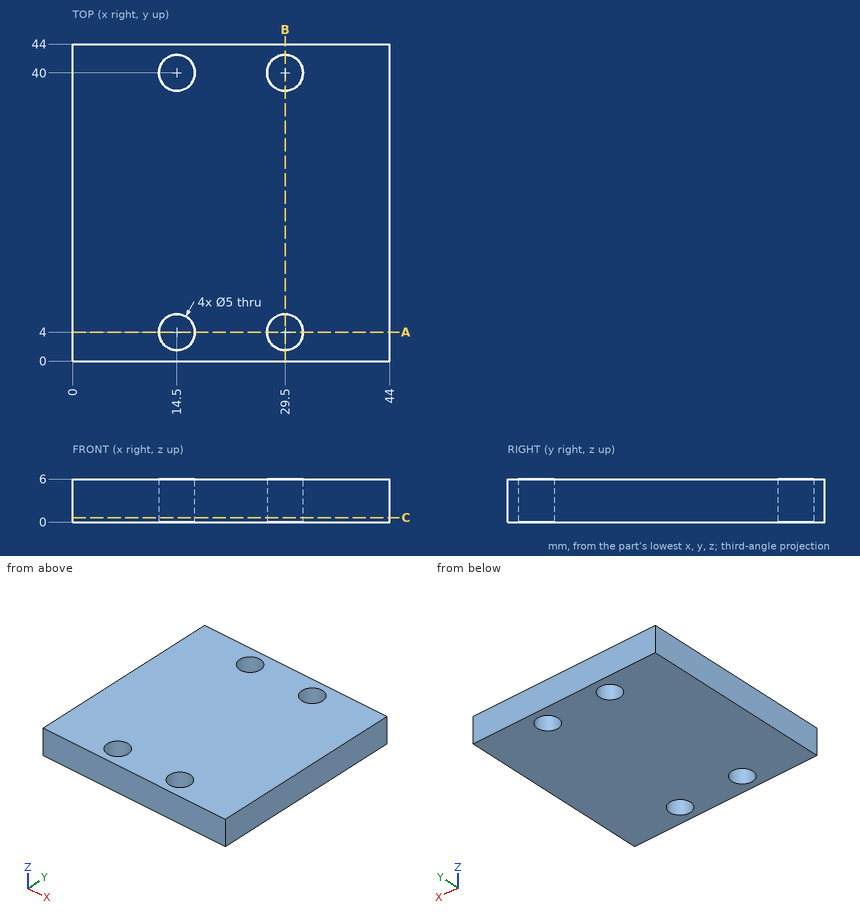
Input: dimensioned drawing with shaded views. Units: mm. Origin: part minimum x, y, z. Round coordinates to 2 decimals unless told otherwise and drop trailing zeros. Order: outer loops, then holes, each group sorted by start corner. A loop starts at its lowest first (then second) coordinate and runs counter-clockwise, first axis right, second up. Notation, with made-up numbers: (-27, 19) -> (31, 19) arc R29 cw to (31, 43) -> close; hole circle Ø5 at (37, 76.5). An arc over 180 degrees is marked (long way). One line per item, written item: value. Start each with the question number.
Q1. Section query C-C (z = 0.65). Return the cut outline in (x, y).
Q2. Section query B-B (x = 29.5). Return the cut outline in (y, z), plus the area to 3 significant figures.
Q3. Section query A-A (y = 4). Return the cut outline in (x, z).
Q4. Material intervals for probe 1 along Y at (x, z) = (14.5, 0.8); probe 2 along X at (y, z) = (4, 3.5); probe 3 along Y at (x, z) = (29, 5.65), sorted ascending.
Findings below:
1. outline: (0, 0) -> (44, 0) -> (44, 44) -> (0, 44) -> close; hole circle Ø5 at (14.5, 4); hole circle Ø5 at (14.5, 40); hole circle Ø5 at (29.5, 4); hole circle Ø5 at (29.5, 40)
2. outline: (0, 0) -> (1.5, 0) -> (1.5, 6) -> (0, 6) -> close; (6.5, 0) -> (37.5, 0) -> (37.5, 6) -> (6.5, 6) -> close; (42.5, 0) -> (44, 0) -> (44, 6) -> (42.5, 6) -> close
2. area: 204 mm²
3. outline: (0, 0) -> (12, 0) -> (12, 6) -> (0, 6) -> close; (17, 0) -> (27, 0) -> (27, 6) -> (17, 6) -> close; (32, 0) -> (44, 0) -> (44, 6) -> (32, 6) -> close
4. probe 1: 0 to 1.5, 6.5 to 37.5, 42.5 to 44
4. probe 2: 0 to 12, 17 to 27, 32 to 44
4. probe 3: 0 to 1.55, 6.45 to 37.55, 42.45 to 44
